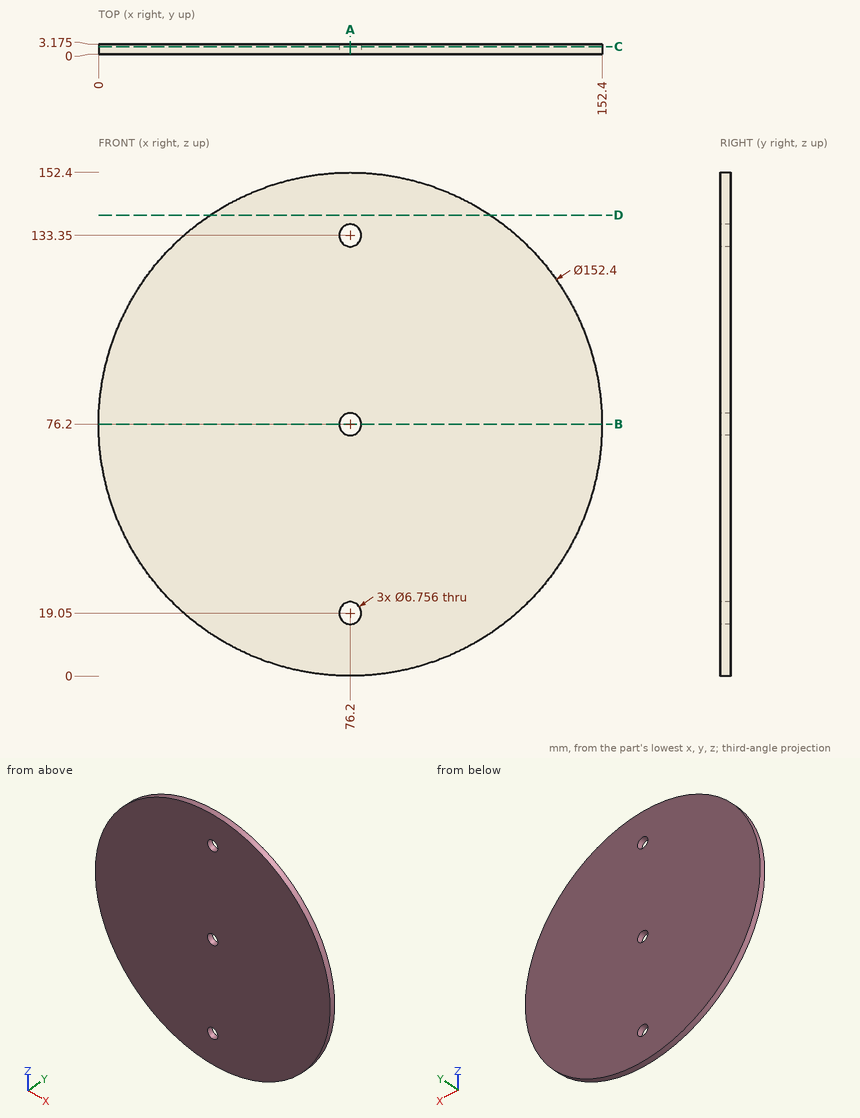
Design review of the part shown in the three views and the two pictorial views. Dimensions are in mm from the part's minimum x, y and z. Coordinates: 2 decimals unless noted, no trailing zeros. Order: outer loops, then holes, each group sorted by start corner. A loop starts at its lowest first (then second) coordinate and runs counter-clockwise, first axis right, second up.
Item 1: Take a section at C-C, the plane y = 2.35. Write out the cut boundary in (x, z).
Item 2: Take a section at B-B, the plane z = 76.2. Write out the cut boundary in (x, y) (1 decimal).
Item 3: For pin 1 Ø5.5 at (x, z) = (76.2, 76.2) entering from +Y, flat-tipped, find the tip position at first contact; note if it passes through.
Item 4: Take a section at A-A, the plane x = 76.2. Write out the cut boundary in (y, z) (1 decimal).
Item 5: For line 1 (Z direction, x = 76.5, y = 0.65) (1 decimal); line 2 (X direction, y = 0.2, z = 79); line 3 (Z direction, x = 115.5, y = 2.95) (1 decimal), list the stretches that pass through material, from the lowest coordinate up.
Item 6: Take a section at D-D, the plane z = 139.5. Write out the cut boundary in (x, y) (1 decimal).
The answers:
1. outline: circle Ø152.4 at (76.2, 76.2); hole circle Ø6.76 at (76.2, 19.05); hole circle Ø6.76 at (76.2, 76.2); hole circle Ø6.76 at (76.2, 133.35)
2. outline: (0, 0) - (72.8, 0) - (72.8, 3.2) - (0, 3.2) - close; (79.6, 0) - (152.4, 0) - (152.4, 3.2) - (79.6, 3.2) - close
3. pin 1: passes through
4. outline: (0, 0) - (3.2, 0) - (3.2, 15.7) - (0, 15.7) - close; (0, 22.4) - (3.2, 22.4) - (3.2, 72.8) - (0, 72.8) - close; (0, 79.6) - (3.2, 79.6) - (3.2, 130) - (0, 130) - close; (0, 136.7) - (3.2, 136.7) - (3.2, 152.4) - (0, 152.4) - close
5. line 1: z = 0 to 15.7, 22.4 to 72.8, 79.6 to 130, 136.7 to 152.4
5. line 2: x = 0.05 to 74.31, 78.09 to 152.35
5. line 3: z = 10.9 to 141.5
6. outline: (33.8, 0) - (118.6, 0) - (118.6, 3.2) - (33.8, 3.2) - close
